Part print with two shaded views. Sizes in mm from the minimum x, y, z corner. Coordinates: 2 decimals unless noted, no trailing zeros. Loops run counter-clockwise (first coordinate to the right, second up) from the corner with the lowest first, then second, coordinate; pieces in that order, holes last.
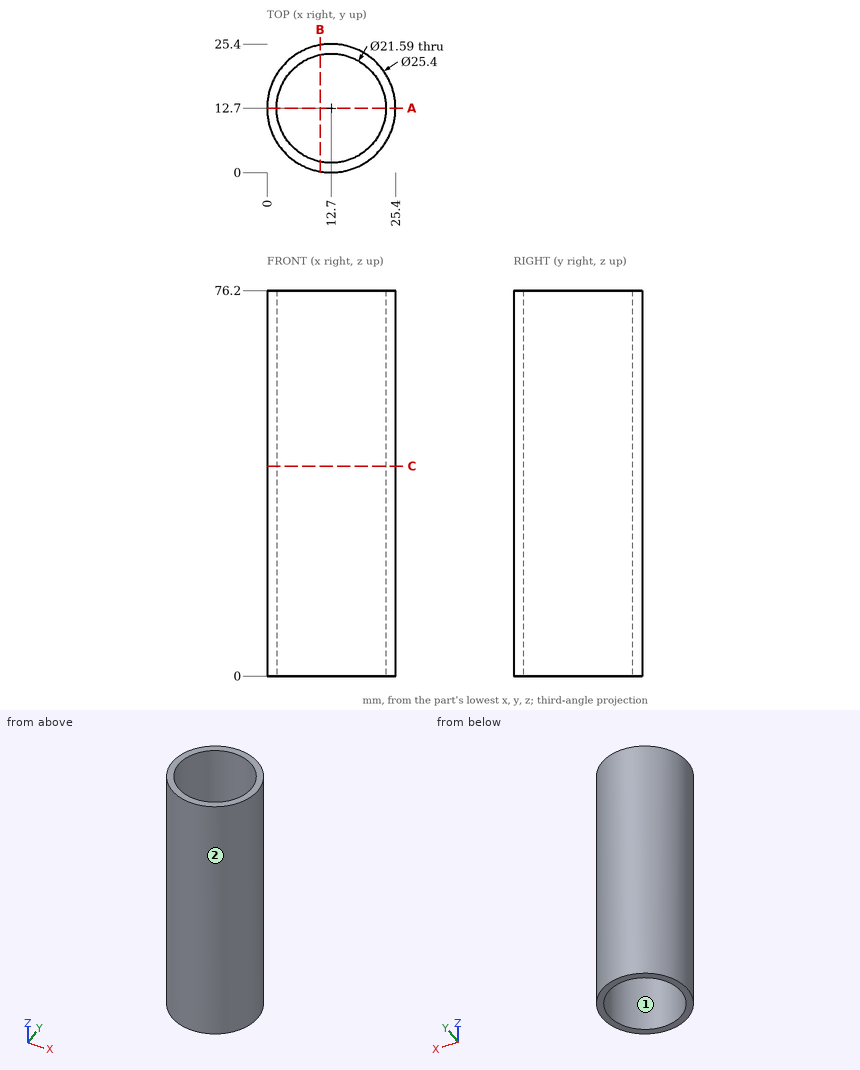
Q1. Slice it at C-C (z = 41.5). List the corners of the cut face in (x, y) (3 decimals).
Answers:
outline: circle Ø25.4 at (12.7, 12.7); hole circle Ø21.59 at (12.7, 12.7)
Q2. Mould opens along Y. For the marked faces 1 and 2 say: +Y half, -Y half, draft (parallel to the pull), parting line (faces both ways), or undercut.
Answers:
face 1: undercut
face 2: parting line
Q3. Slice it at A-A (y = 12.7). List the corners of the cut face in (x, z) (3 decimals), and give its area (3 significant figures).
Answers:
outline: (0, 0) - (1.905, 0) - (1.905, 76.2) - (0, 76.2) - close; (23.495, 0) - (25.4, 0) - (25.4, 76.2) - (23.495, 76.2) - close
area: 290 mm2
Q4. Drill centre lines: line 1 (Y direction, x = 12.7, z = 53) (3 decimals); line 2 (X direction, y = 12.5, z = 48.5); line 3 (X direction, y = 21.75, z = 51.5). Where is each one in solid material? Low to high.
Answers:
line 1: y = 0 to 1.905, 23.495 to 25.4
line 2: x = 0 to 1.91, 23.49 to 25.4
line 3: x = 3.79 to 6.82, 18.58 to 21.61
Q5. Flat gauge pins, fed straight in: P1, Ø5, axis at y = 6, z = 39, coming from the -X side; P2, Ø10, axis at y = 9.5, z = 39, coming from the +X side; P3, Ø2, axis at x = 9, z = 36, coming from the +Y side; P4, Ø12, axis at x = 4.5, z = 28.5, coming from the -Y side. Where does each tip first touch, or does it go through?
Answers:
P1: stops at x = 0.71
P2: stops at x = 25.4
P3: stops at y = 25.11
P4: stops at y = 0.19
Q6. Slice it at B-B (x = 10.5). List the corners of the cut face in (y, z).
Answers:
outline: (0.19, 0) - (2.13, 0) - (2.13, 76.2) - (0.19, 76.2) - close; (23.27, 0) - (25.21, 0) - (25.21, 76.2) - (23.27, 76.2) - close
